The model under review builds one solid part; all positions refer to its coordinate system, in mm. Face numbers are marked on the shaded views. A direction names the side the tool comes from. Coordinates: 2 decimals unless noted, no trailing zeros. Write each loop counter-clockwise with the first axis right and the second up, starting at its lowest first coordinate (ties: lowest second). Pieces come first, ordered by that corner, then holes. Notation, with made-up numbers: M -8.5,58 L 8.5,58 A14 ccw 8.5,73 Z; hole C -7.75,72 d1. An arc over 180 degrees is marked long. Answer as a JSON object with one key per item and string values.
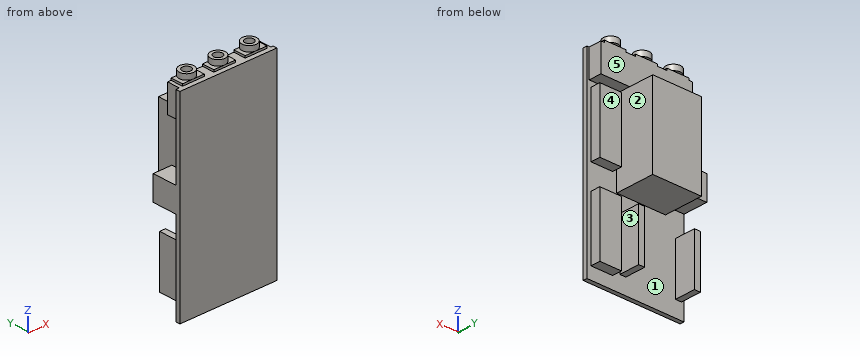
```python
from build123d import *

# Parameters (mm, degrees)
SKETCH1_W           = 39.8
SKETCH1_H           = 79.8
BOSS_EXTRUDE1_DEPTH = 1.7
SKETCH2_W           = 20
SKETCH2_H           = 34.2
BOSS_EXTRUDE2_DEPTH = 15.9
SKETCH3_W           = 2.45
SKETCH3_H           = 20.9
BOSS_EXTRUDE3_DEPTH = 8.35
SKETCH4_W           = 7.63
SKETCH4_H           = 9.9
BOSS_EXTRUDE4_DEPTH = 10.05
SKETCH5_W           = 8.9
SKETCH5_H           = 25.6
BOSS_EXTRUDE5_DEPTH = 3.9
SKETCH6_W           = 37.52
SKETCH6_H           = 11.3
BOSS_EXTRUDE6_DEPTH = 5.16
SKETCH7_W           = 8.95
SKETCH7_H           = 5
BOSS_EXTRUDE7_DEPTH = 0.82
SKETCH8_R           = 3
SKETCH8_R_2         = 1.775
BOSS_EXTRUDE8_DEPTH = 2.22
LPATTERN1_COUNT     = 2
LPATTERN1_PITCH     = 12.875
LPATTERN2_COUNT     = 2
LPATTERN2_PITCH     = 12.875


with BuildPart() as part:
    # Sketch1 → Boss-Extrude1 (new body)
    with BuildSketch(Plane(origin=(0, 0, 0), x_dir=(1, 0, 0), z_dir=(0, 1, 0))):
        Rectangle(SKETCH1_W, SKETCH1_H)
    extrude(amount=BOSS_EXTRUDE1_DEPTH)

    # Sketch2 → Boss-Extrude2 (add)
    with BuildSketch(Plane(origin=(0, 1.7, 0), x_dir=(1, 0, 0), z_dir=(0, 1, 0))):
        with Locations((-2.27, -11.08)):
            Rectangle(SKETCH2_W, SKETCH2_H)
    extrude(amount=BOSS_EXTRUDE2_DEPTH)

    # Sketch3 → Boss-Extrude3 (add)
    with BuildSketch(Plane(origin=(0, 1.7, 0), x_dir=(1, 0, 0), z_dir=(0, 1, 0))):
        with Locations((-17.615, 23)):
            Rectangle(SKETCH3_W, SKETCH3_H)
        with Locations((5.235, 23)):
            Rectangle(SKETCH3_W, SKETCH3_H)
    extrude(amount=BOSS_EXTRUDE3_DEPTH)

    # Sketch4 → Boss-Extrude4 (add)
    with BuildSketch(Plane(origin=(0, 1.7, 0), x_dir=(1, 0, 0), z_dir=(0, 1, 0))):
        with Locations((-16.085, -2.05)):
            Rectangle(SKETCH4_W, SKETCH4_H)
    extrude(amount=BOSS_EXTRUDE4_DEPTH)

    # Sketch5 → Boss-Extrude5 (add)
    with BuildSketch(Plane(origin=(0, 1.7, 0), x_dir=(1, 0, 0), z_dir=(0, 1, 0))):
        with Locations((13.85, -13.55)):
            Rectangle(SKETCH5_W, SKETCH5_H)
        with Locations((13.85, 22.15)):
            Rectangle(SKETCH5_W, SKETCH5_H)
    extrude(amount=BOSS_EXTRUDE5_DEPTH)

    # Sketch6 → Boss-Extrude6 (add)
    with BuildSketch(Plane(origin=(0, 1.7, 0), x_dir=(1, 0, 0), z_dir=(0, 1, 0))):
        with Locations((0.26, -34.25)):
            Rectangle(SKETCH6_W, SKETCH6_H)
    extrude(amount=BOSS_EXTRUDE6_DEPTH)

    # Sketch7 → Boss-Extrude7 (add)
    with BuildSketch(Plane.XY.offset(39.9)):
        with Locations((0.26, 4.36)):
            Rectangle(SKETCH7_W, SKETCH7_H)
    boss_extrude7 = extrude(amount=BOSS_EXTRUDE7_DEPTH)

    # Sketch8 → Boss-Extrude8 (add)
    with BuildSketch(Plane.XY.offset(40.72)):
        with Locations((0.26, 4.86)):
            Circle(SKETCH8_R)
        with Locations((0.26, 4.86)):
            Circle(SKETCH8_R_2, mode=Mode.SUBTRACT)
    boss_extrude8 = extrude(amount=BOSS_EXTRUDE8_DEPTH)

    # LPattern1: Boss-Extrude7, Boss-Extrude8 ×2
    with Locations(*[(-i * LPATTERN1_PITCH, 0, 0) for i in range(1, LPATTERN1_COUNT)]):
        add(boss_extrude7)
        add(boss_extrude8)

    # LPattern2: Boss-Extrude7, Boss-Extrude8 ×2
    with Locations(*[(i * LPATTERN2_PITCH, 0, 0) for i in range(1, LPATTERN2_COUNT)]):
        add(boss_extrude7)
        add(boss_extrude8)


solid = part.part
```
(1) Draft analysis for pull direction Z (two halves, no side actions). For the marked faces 1 and 2, state which applies: released by +Z, released by -Z, zero draft, split by the parting line, or undercut.
Results list:
{"face 1": "undercut", "face 2": "zero draft"}
(2) Wall thickness on line 1 along X through (y, z) = (3.75, -14); line 2 along Z through (x, y) = (5.5, 7); line 3 along Z through (x, y) = (-10, 5): over which ranges is each line inside the solid? List them lowest first. Write a range as from..to.
Results list:
{"line 1": "-18.84..-16.39, 4.01..6.46, 9.4..18.3", "line 2": "-33.45..-12.55, -6.02..28.18", "line 3": "-6.02..28.18, 28.6..42.94"}
(3) For pin 1 Ø10 at (y, z) = (10.5, -3) entering from +X; pin 2 Ø2.5 at (x, z) = (5, -26) entering from +Y; pin 3 Ø5 at (x, y) = (-6.5, 9) entering from +Z, all flat-tipped, find the tip position at first contact; note any pin that passes through.
Results list:
{"pin 1": "x = 7.73", "pin 2": "y = 10.05", "pin 3": "z = 39.9"}
(4) For the marked faces 3, 4 and 5, list the 3-axis set-ups (+Z, -Z, +X, -X, +Y, -Y) from which the entire face can be reached by the end or side of a thin tool; tool diameter is ignored.
Results list:
{"face 3": "-Z, +Y", "face 4": "-Z, +X, +Y", "face 5": "+X, -X, +Y"}
(5) Add section B-B on z = -2. Give the boundary of the cut face in (x, y), and give its area (3 significant figures).
Results list:
{"outline": "M -19.9,0 L 19.9,0 L 19.9,1.7 L 7.73,1.7 L 7.73,17.6 L -12.27,17.6 L -12.27,11.75 L -19.9,11.75 Z", "area": "462 mm²"}
(6) Add section A-A on y = 9. Give the boundary of the cut face in (x, z), and give its area (3 significant figures).
Results list:
{"outline": "M -19.9,-2.9 L -12.27,-2.9 L -12.27,-6.02 L 7.73,-6.02 L 7.73,28.18 L -12.27,28.18 L -12.27,7 L -19.9,7 Z; M -18.84,-33.45 L -16.39,-33.45 L -16.39,-12.55 L -18.84,-12.55 Z; M 4.01,-33.45 L 6.46,-33.45 L 6.46,-12.55 L 4.01,-12.55 Z", "area": "862 mm²"}
(7) Add section C-C on z = -24. Give the boundary of the cut face in (x, y).
Results list:
{"outline": "M -19.9,0 L 19.9,0 L 19.9,1.7 L 18.3,1.7 L 18.3,5.6 L 9.4,5.6 L 9.4,1.7 L 6.46,1.7 L 6.46,10.05 L 4.01,10.05 L 4.01,1.7 L -16.39,1.7 L -16.39,10.05 L -18.84,10.05 L -18.84,1.7 L -19.9,1.7 Z"}
